from build123d import *

# Parameters (mm, degrees)
F0_R     = 2.75
F1_DEPTH = 15
F2_R     = 2.75
F3_DEPTH = 22
F4_R     = 2.75
F5_DEPTH = 10


with BuildPart() as f1:
    # F0 (on Top) → F1 (new body)
    with BuildSketch(Plane.XY):
        Polygon((20, -5), (20, 5), (5, 5), (5, 20), (-5, 20), (-5, 5), (-20, 5), (-20, -5), (-5, -5), (-5, -20), (5, -20), (5, -5), align=None)
        with Locations((0, -15)):
            Circle(F0_R, mode=Mode.SUBTRACT)
        with BuildLine():
            ThreePointArc((2.079062, 1.8), (0, -2.75), (-2.079062, 1.8))
            Line((-2.079062, 1.8), (2.079062, 1.8))
        make_face(mode=Mode.SUBTRACT)
        with Locations((-15, 0)):
            Circle(F0_R, mode=Mode.SUBTRACT)
        with Locations((15, 0)):
            Circle(F0_R, mode=Mode.SUBTRACT)
        with Locations((0, 15)):
            Circle(F0_R, mode=Mode.SUBTRACT)
    extrude(amount=F1_DEPTH)

    # F2 (on Top) → F3 (join)
    with BuildSketch(Plane.XY):
        with Locations((0, 15)):
            Circle(F2_R)
        with Locations((15, 0)):
            Circle(F2_R)
        with Locations((0, -15)):
            Circle(F2_R)
        with Locations((-15, 0)):
            Circle(F2_R)
    extrude(amount=F3_DEPTH)

    # F4 (on face) → F5 (join)
    with BuildSketch(Plane.XY.offset(22)):
        with Locations((0, 15)):
            Circle(F4_R)
    extrude(amount=F5_DEPTH)


solid = f1.part
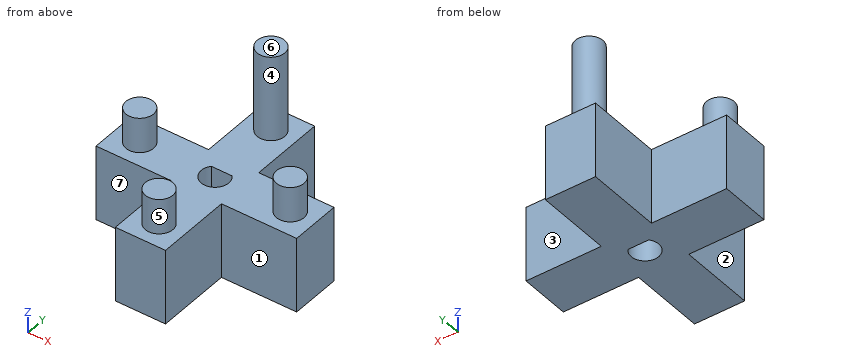
Build history of the part. All positions in model axes, mm. Face numbers are marked on the shaded views. A direction names the side the tool comes from. Coordinates: 2 decimals unless noted, no trailing zeros. Order: outer loops, then holes, each group sorted by start corner. A loop starts at its lowest first (then second) coordinate and runs counter-clockwise, first axis right, second up. Notation, with made-up numbers: (-15.5, -4) -> (-10.5, -4) arc R22 ccw to (-10.5, 7) -> close; hole circle Ø5 at (58, 71.25). An arc over 180 degrees is marked (long way). One line per item, written item: value.
(1) Tool access for the marked faces 1, 2, 3 and 4: list every direction of +Z, -Z, +X, -X, +Y, -Y with a clear straight run to the whole face (end or side of a thin tool).
Checked values:
face 1: +Z, -Z, +X, -Y
face 2: +Z, -Z, -X, -Y
face 3: +Z, -Z, +X, +Y
face 4: +Z
(2) Slice it at D-D, the plane z = 19. List the corners of the cut face in (x, y), plus the area to 3 significant figures.
Checked values:
outline: circle Ø5.5 at (-15, 0); circle Ø5.5 at (0, -15); circle Ø5.5 at (0, 15); circle Ø5.5 at (15, 0)
area: 95.0 mm2
(3) Probe line 1 (X direction, y = 0, z = 9.5); line 2 (Y direction, x = 0, z = 11); line 3 (Z direction, x = -5.5, y = -3.5). List the from-to ranges inside material, lowest first. Write a range as [from, to].
Checked values:
line 1: [-20, -2.75], [2.75, 20]
line 2: [-20, -2.75], [1.8, 20]
line 3: [0, 15]
(4) Slice it at B-B, the plane y = 15. List the corners of the cut face in (x, z).
Checked values:
outline: (-5, 0) -> (5, 0) -> (5, 15) -> (2.75, 15) -> (2.75, 32) -> (-2.75, 32) -> (-2.75, 15) -> (-5, 15) -> close
(5) Slice it at A-A, the plane x = 0. List the corners of the cut face in (y, z).
Checked values:
outline: (-20, 0) -> (-2.75, 0) -> (-2.75, 15) -> (-12.25, 15) -> (-12.25, 22) -> (-17.75, 22) -> (-17.75, 15) -> (-20, 15) -> close; (1.8, 0) -> (20, 0) -> (20, 15) -> (17.75, 15) -> (17.75, 32) -> (12.25, 32) -> (12.25, 15) -> (1.8, 15) -> close
(6) Mould opens along Y. For the marked faces 5, 6 and 7 say: pulls with the +Y half, pulls with the -Y half, needs draft (parallel to the pull), parting line crosses it, or undercut.
Checked values:
face 5: undercut
face 6: needs draft
face 7: pulls with the -Y half
(7) Drop flat-ended pins along their axis: pin 1 Ø16.5 at (y, z) = (15, 9) entering from +X; pin 2 Ø12 at (x, z) = (-12.5, 8) entering from +Y; pin 3 Ø3 at (x, y) = (-14.5, 1) entering from +Z; pin 4 Ø5 at (x, y) = (12, -9) entering from -Z. Give the stop position or say it passes through.
Checked values:
pin 1: x = 5
pin 2: y = 5
pin 3: z = 22
pin 4: through
(8) Slice it at C-C, the plane x = 15. List the corners of the cut face in (y, z), plus the area to 4 significant figures.
Checked values:
outline: (-5, 0) -> (5, 0) -> (5, 15) -> (2.75, 15) -> (2.75, 22) -> (-2.75, 22) -> (-2.75, 15) -> (-5, 15) -> close
area: 188.5 mm2
